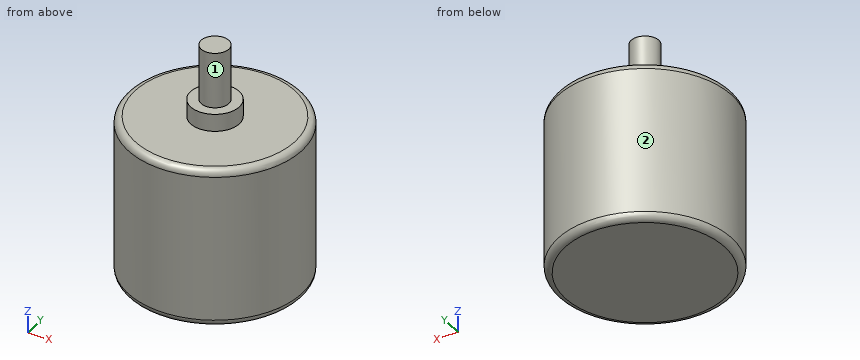
```python
from build123d import *

# Parameters (mm, degrees)
ESBO_O1_R                = 12.5
RESSALTO_EXTRUS_O1_DEPTH = 23
ESBO_O2_R                = 3.5
RESSALTO_EXTRUS_O2_DEPTH = 2.5
FILETE1_R                = 1
ESBO_O3_R                = 2
RESSALTO_EXTRUS_O3_DEPTH = 8


with BuildPart() as part:
    # Esboço1 → Ressalto-extrusão1 (new body)
    with BuildSketch(Plane.XY):
        Circle(ESBO_O1_R)
    extrude(amount=RESSALTO_EXTRUS_O1_DEPTH)

    # Esboço2 → Ressalto-extrusão2 (add)
    with BuildSketch(Plane.XY.offset(23)):
        Circle(ESBO_O2_R)
    extrude(amount=RESSALTO_EXTRUS_O2_DEPTH)

    # Filete1
    filete1_edges = [part.edges().sort_by_distance(p)[0] for p in [
        (-12.5, 0, 0),
        (-12.5, 0, 23),
    ]]
    fillet(filete1_edges, radius=FILETE1_R)

    # Esboço3 → Ressalto-extrusão3 (add)
    with BuildSketch(Plane.XY.offset(25.5)):
        Circle(ESBO_O3_R)
    extrude(amount=RESSALTO_EXTRUS_O3_DEPTH)


solid = part.part
```
Work out the finished part from the listing and answer in its coordinate system (mm). Face numbers are marked on the shaded views. A direction names the side the tool comes from. Coordinates: 2 decimals unless noted, no trailing zeros. Order: outer loops, then holes, each group sorted by start corner. A loop starts at its lowest first (then second) coordinate and runs counter-clockwise, first axis right, second up. Notation, with made-up numbers: (68, -36.75) - (97, -36.75) arc R21 ccw to (97, -3.75) - close; hole circle Ø6 at (-12.5, 69.5). An arc over 180 degrees is marked (long way). Answer as a JSON object with one key per item and string values.
1. Find section A-A on x = 0. Determine the outline of the cut face in (y, z), plus the area to 3 significant figures.
Output values:
{"outline": "(-12.5, 1) arc R1 ccw to (-11.5, 0) - (11.5, 0) arc R1 ccw to (12.5, 1) - (12.5, 22) arc R1 ccw to (11.5, 23) - (3.5, 23) - (3.5, 25.5) - (2, 25.5) - (2, 33.5) - (-2, 33.5) - (-2, 25.5) - (-3.5, 25.5) - (-3.5, 23) - (-11.5, 23) arc R1 ccw to (-12.5, 22) - close", "area": "624 mm²"}
2. Each of these flat-tipped pins is pushed along its axis until it touches: P1, Ø3, axis at x = -5, y = 6.5, coming from the +Z side; P2, Ø5, axis at y = -8.5, z = 26.5, coming from the -X side; P3, Ø10, axis at y = 7, z = 20.5, coming from the -X side; P4, Ø8, axis at x = 10, z = 16, coming from the -Y side. Where does it stop, or does it pass through?
Output values:
{"P1": "stops at z = 23", "P2": "passes through", "P3": "stops at x = -12.34", "P4": "stops at y = -10.97"}
3. Consider line 1 (Y direction, x = -0.25, z = 5.5); line 2 (Z direction, x = 5, y = 7.75); line 3 (X direction, y = -0.25, z = 24.5). Determine where each line is inside the solid, lowest interval first.
Output values:
{"line 1": "y = -12.5 to 12.5", "line 2": "z = 0 to 23", "line 3": "x = -3.49 to 3.49"}
4. Find section D-D on z = 15.5. Determine the outline of the cut face in (x, y).
Output values:
{"outline": "circle Ø25 at (0, 0)"}
5. Find section C-C on z = 26. Determine the outline of the cut face in (x, y).
Output values:
{"outline": "circle Ø4 at (0, 0)"}
6. A tool of negligible diameter and unlimited length cuts with its end or side. For the marked faces 1 and 2, from which of +Z, -Z, +X, -X, +Y, -Y can it reach the whole face along a straight path? Write none if from no direction.
Output values:
{"face 1": "+Z", "face 2": "+Z, -Z"}
